Source: CAD feature listing. Evaluate the final solid. Frame: model axes, mm. Give positions to 0.01 mm unless a question says otherwise; leave off trailing zeros. Order: outer loops, then holes, each group sorted by start corner. A loop starts at its lowest first (then second) coordinate and runs counter-clockwise, first axis right, second up.
Autodesk Inventor part; units mm, degrees
ref_plane "YZ Plane" through (0, 0, 0) normal (1, 0, 0) x (0, 1, 0)
ref_plane "XZ Plane" through (0, 0, 0) normal (0, 1, 0) x (-1, 0, 0)
ref_plane "XY Plane" through (0, 0, 0) normal (0, 0, 1) x (1, 0, 0)
sketch "main" plane through (0, 0, 0) normal (0, 0, 1) x (1, 0, 0)
  circle A0 centre (10.1168, 23.8511) radius 4.064
  circle A1 centre (10.1168, 11.1511) radius 4.064
  circle A2 centre (10.1168, -14.2489) radius 4.064
  circle A3 centre (16.4668, -33.2989) radius 4.0005
  circle A4 centre (16.4668, -58.6989) radius 4.0005
  circle A5 centre (10.1168, -77.7489) radius 4.064
  circle A6 centre (3.7668, 169.9011) radius 2.1844
  circle A7 centre (16.4668, 169.9011) radius 2.1844
  circle A8 centre (10.1168, -103.1489) radius 4.064
  circle A9 centre (16.4668, -122.1989) radius 4.0005
  circle A10 centre (3.7668, -172.9989) radius 2.1844
  circle A11 centre (16.4668, -172.9989) radius 2.1844
  line L0 (-20.0457, 131.4398) -> (-20.0457, -168.0589)
  line L1 (22.8168, -185.6989) -> (22.8168, 182.6011)
  line L2 (-16.7075, -176.6406) -> (-6.3583, -187.9307)
  line L3 (3.0036, -192.0489) -> (16.4668, -192.0489)
  arc A12 (-20.0457, -168.0589) -> (-16.7075, -176.6406) centre (-7.3457, -168.0589) ccw
  arc A13 (-6.3583, -187.9307) -> (3.0036, -192.0489) centre (3.0036, -179.3489) ccw
  circle A14 centre (16.4668, -147.5989) radius 4.0005
  arc A15 (16.4668, -192.0489) -> (22.8168, -185.6989) centre (16.4668, -185.6989) ccw
  line L4 (16.4668, 188.9511) -> (2.0773, 188.9511)
  line L5 (-3.9805, 184.505) -> (-19.4614, 135.2476)
  arc A16 (-19.4614, 135.2476) -> (-20.0457, 131.4398) centre (-7.3457, 131.4398) ccw
  circle A17 centre (10.1168, 49.2511) radius 4.064
  circle A18 centre (10.1168, 61.9511) radius 4.064
  circle A19 centre (10.1168, 87.3511) radius 4.064
  circle A20 centre (16.4668, 106.4011) radius 4.0005
  circle A21 centre (16.4668, 131.8011) radius 4.0005
  arc A22 (22.8168, 182.6011) -> (16.4668, 188.9511) centre (16.4668, 182.6011) ccw
  arc A23 (2.0773, 188.9511) -> (-3.9805, 184.505) centre (2.0773, 182.6011) ccw
  circle A24 centre (16.4668, 119.1011) radius 4.0005
  circle A25 centre (16.4668, -45.9989) radius 4.0005
  circle A26 centre (16.4668, -134.8989) radius 4.0005
  point P0 (5.8318, -6.3003)
  dimension "d16" = 12.7
  dimension "d17" = 6.35
  dimension "d18" = 6.35
  dimension "d19" = 8.001
  dimension "d20" = 25.4
  dimension "d21" = 165.1
  dimension "d22" = 254
  dimension "d23" = 8.128
  dimension "d24" = 25.4
  dimension "d25" = 38.1
  dimension "d26" = 25.4
sketch "Sketch1" plane through (0, 0, 0) normal (1, 0, 0) x (0, 1, 0)
  circle A0 centre (6.35, -146.05) radius 4.064
  circle A1 centre (6.35, -158.75) radius 4.064
  circle A2 centre (6.35, -184.15) radius 4.064
  circle A3 centre (12.7, -203.2) radius 4.0005
  circle A4 centre (12.7, -228.6) radius 4.0005
  circle A5 centre (6.35, -247.65) radius 4.064
  circle A6 centre (0, 0) radius 2.1844
  circle A7 centre (12.7, 0) radius 2.1844
  circle A8 centre (6.35, -273.05) radius 4.064
  circle A9 centre (12.7, -292.1) radius 4.0005
  circle A10 centre (0, -342.9) radius 2.1844
  circle A11 centre (12.7, -342.9) radius 2.1844
  line L0 (-23.8125, -38.4612) -> (-23.8125, -337.9599)
  line L1 (19.05, -355.6) -> (19.05, 12.7)
  line L2 (-20.4744, -346.5416) -> (-10.1251, -357.8317)
  line L3 (-0.7632, -361.95) -> (12.7, -361.95)
  arc A12 (-23.8125, -337.9599) -> (-20.4744, -346.5416) centre (-11.1125, -337.9599) ccw
  arc A13 (-10.1251, -357.8317) -> (-0.7632, -361.95) centre (-0.7632, -349.25) ccw
  circle A14 centre (12.7, -317.5) radius 4.0005
  arc A15 (12.7, -361.95) -> (19.05, -355.6) centre (12.7, -355.6) ccw
  line L4 (12.7, 19.05) -> (-1.6895, 19.05)
  line L5 (-7.7473, 14.6039) -> (-23.2282, -34.6534)
  arc A16 (-23.2282, -34.6534) -> (-23.8125, -38.4612) centre (-11.1125, -38.4612) ccw
  circle A17 centre (6.35, -120.65) radius 4.064
  circle A18 centre (6.35, -107.95) radius 4.064
  circle A19 centre (6.35, -82.55) radius 4.064
  circle A20 centre (12.7, -63.5) radius 4.0005
  circle A21 centre (12.7, -38.1) radius 4.0005
  arc A22 (19.05, 12.7) -> (12.7, 19.05) centre (12.7, 12.7) ccw
  arc A23 (-1.6895, 19.05) -> (-7.7473, 14.6039) centre (-1.6895, 12.7) ccw
  circle A24 centre (12.7, -50.8) radius 4.0005
  circle A25 centre (12.7, -215.9) radius 4.0005
  circle A26 centre (12.7, -304.8) radius 4.0005
extrude "Extrusion1" add sketch "Sketch1" along normal blind 1.5875
properties part number "Skirt" material "Acetal Resin, White"
1) Section query C-C on z = -304.8. Output: boundary loops of the cut face in (x, y), and give its area (3 significant figures).
Checks:
outline: (0, -23.81) - (1.59, -23.81) - (1.59, 8.7) - (0, 8.7) - close; (0, 16.7) - (1.59, 16.7) - (1.59, 19.05) - (0, 19.05) - close
area: 55.3 mm2
2) Section query D-D on z = -31. Output: boundary loops of the cut face in (x, y).
Checks:
outline: (0, -22.08) - (1.59, -22.08) - (1.59, 19.05) - (0, 19.05) - close
3) Section query B-B on x = 1.3. State how many separate pieces and enclosed holes the cut face has, and give its area (3 significant figures).
Checks:
separate pieces: 1
enclosed holes: 21
area: 14,700 mm2
4) First-contact query: pin 1 Ø4 at (y, z) = (-8, -184.5) entering from -X; pin 2 Ø6.5 at (y, z) = (12.7, -215.9) entering from -X. Flat tips, straight axial feed; report the tip coordinate or a pass-through.
Checks:
pin 1: stops at x = 0
pin 2: passes through
5) Pull-direction query (Y, two-part tool) for faces 1 (the face through (0.78, -15.37, -352.11)), 2 (the face through (0.783, 12.179, -321.466)), 3 (the face through (0.78, 17.14, 17.24)); classes: +Y half, -Y half, draft (parallel to the pull), parting line (faces both ways), or undercut.
Checks:
face 1: -Y half
face 2: undercut
face 3: +Y half
6) Ray query, L1, parallel to Y at x = 0.25, z = -184; L2, parallel to Z at x = 1.2, y = -1; L3, parallel to Y at x = 0.1, z = -38.5. Return the intervals inside material, ascending.
Checks:
L1: y = -23.81 to 2.29, 10.41 to 19.05
L2: z = -361.95 to -344.84, -340.96 to -1.94, 1.94 to 19.05
L3: y = -23.81 to 8.72, 16.68 to 19.05
7) Section query A-A on z = -82.55. Output: boundary loops of the cut face in (x, y).
Checks:
outline: (0, -23.81) - (1.59, -23.81) - (1.59, 2.29) - (0, 2.29) - close; (0, 10.41) - (1.59, 10.41) - (1.59, 19.05) - (0, 19.05) - close
